Input: part model. Units: mm. Frame: model coordinates. Round coordinates to 2 decimals unless told otherwise and drop trailing zeros. Loops run counter-clockwise (first coordinate to the right, second up) from the corner with the lowest first, then second, coordinate; pieces in that order, holes last. Notation, with made-up numbers: M -26.5,33 L 24.5,33 A28 cw 24.5,52 Z; hole C -8.75,75.25 d10. An arc over 180 degrees is marked long. Put each result on its own line as item: value. Start each with the question number.
1) Section B-B on z = -2.5. Output: boundary loops of the cut face in (x, y), plus the area to 3 significant figures.
2) Section C-C on y = 5. Output: boundary loops of the cut face in (x, z), plus the area to 3 significant figures.
3) Section D-D on z = -8.75. Output: boundary loops of the cut face in (x, y), plus the area to 3 significant figures.
4) Line query: probe 1 along X at (y, z) = (5, -6.75); probe 2 along X at (y, z) = (5, -3); probe 3 along X at (y, z) = (5, -2). Output: solid intervals per line, ascending.
5) Pin query (flat end, axial travel): pin 1 (2.5 mm diameter, centred on x = -10, y = 5, fed in from -Z). Return the tip coordinate at first contact, or that it passes through.
6) Draft query along X for faces 1 (the face through (0, 10, -6)), 2 (the face through (15, 5, -5)), 3 (the face through (8.9, 6.19, -5.07)). Return one class per face: +X half, -X half, draft (parallel to the pull), parting line (faces both ways), or undercut.
7) Section A-A on x = -10. Output: boundary loops of the cut face in (y, z).
Autodesk Inventor part; units mm, degrees
ref_plane "YZ Plane" through (0, 0, 0) normal (1, 0, 0) x (0, 1, 0)
ref_plane "XZ Plane" through (0, 0, 0) normal (0, 1, 0) x (-1, 0, 0)
ref_plane "XY Plane" through (0, 0, 0) normal (0, 0, 1) x (1, 0, 0)
sketch "Sketch2" plane through (0, 0, 0) normal (0, 1, 0) x (-1, 0, 0)
  line L0 (5, 0) -> (15, 0)
  line L1 (15, 0) -> (15, -10)
  line L2 (15, -10) -> (-15, -10)
  line L3 (-15, -10) -> (-15, 0)
  line L4 (-15, 0) -> (-5, 0)
  arc A0 (-5, 0) -> (5, 0) centre (0, 0) ccw
  dimension "d0" = 10
  dimension "d1" = 5
  dimension "d12" = 10
extrude "Extrusion1" add sketch "Sketch2" along normal blind 10
sketch "Sketch3" plane through (0, 0, 0) normal (0, 0, 1) x (1, 0, 0)
  line L0 (5, 0) -> (15, 0) construction
  line L1 (15, 0) -> (15, 10) construction
  line L2 (5, 10) -> (15, 10) construction
  line L3 (5, 0) -> (5, 10) construction
  line L4 (-15, 0) -> (-5, 0) construction
  line L5 (-5, 0) -> (-5, 10) construction
  line L6 (-15, 10) -> (-5, 10) construction
  line L7 (-15, 0) -> (-15, 10) construction
  line L8 (15, 10) -> (5, 0) construction
  line L9 (5, 10) -> (15, 0) construction
  line L10 (-5, 0) -> (-15, 10) construction
  line L11 (-5, 10) -> (-15, 0) construction
  point P0 (0, 0)
  point P1 (-10, 5)
  point P2 (10, 5)
hole "Hole1" at (-10, 5, 0) at (10, 5, 0) direction (0, 0, -1) diameter 3.242 end through all
properties part number "P014-Chapeau_bielle"
Geometry results:
1. outline: M -15,0 L -4.33,0 L -4.33,10 L -15,10 Z; M 4.33,0 L 15,0 L 15,10 L 4.33,10 Z; hole C -10,5 d3.24; hole C 10,5 d3.24
1. area: 197 mm²
2. outline: M -15,-10 L -11.62,-10 L -11.62,0 L -15,0 Z; M -8.38,-10 L 8.38,-10 L 8.38,0 L 5,0 A5 cw -5,0 L -8.38,0 Z; M 11.62,-10 L 15,-10 L 15,0 L 11.62,0 Z
2. area: 196 mm²
3. outline: M -15,0 L 15,0 L 15,10 L -15,10 Z; hole C -10,5 d3.24; hole C 10,5 d3.24
3. area: 283 mm²
4. probe 1: x = -15 to -11.62, -8.38 to 8.38, 11.62 to 15
4. probe 2: x = -15 to -11.62, -8.38 to -4, 4 to 8.38, 11.62 to 15
4. probe 3: x = -15 to -11.62, -8.38 to -4.58, 4.58 to 8.38, 11.62 to 15
5. pin 1: passes through
6. face 1: draft
6. face 2: +X half
6. face 3: undercut
7. outline: M 0,-10 L 3.38,-10 L 3.38,0 L 0,0 Z; M 6.62,-10 L 10,-10 L 10,0 L 6.62,0 Z
